Input: part model. Units: mm. Frame: model coordinates. Face numbers are marked on the shaded views. A direction names the side the tool comes from. Round coordinates to 2 decimals unless told otherwise and drop trailing zeros. Loops run counter-clockwise (first coordinate to the right, second up) from the corner with the lowest first, then second, coordinate; pieces in that order, holes last. Notation, with made-up numbers: (-3.75, 25.5) -> (24.25, 25.5) arc R24 cw to (24.25, 50.5) -> close; hole circle Ø10 at (-25.75, -5.5). An arc over 180 degrees is marked (long way). Answer as a JSON object with one key per item and string values.
```python
from build123d import *

# Parameters (mm, degrees)
F1_DEPTH = 5
F2_W     = 160
F2_H     = 2.5
F3_DEPTH = 25
F4_W     = 35
F4_H     = 30
F5_DEPTH = 4
F6_W     = 35
F6_H     = 30
F7_DEPTH = 4
F8_W     = 168
F8_H     = 35
F9_DEPTH = 4


with BuildPart() as f1:
    # F0 (on Top) → F1 (new body)
    with BuildSketch(Plane.XY):
        with BuildLine():
            Line((-60.891874, 20), (-60.891874, 0))
            Line((-60.891874, 0), (-60.891874, -15))
            Line((-60.891874, -15), (99.108126, -15))
            Line((99.108126, -15), (99.108126, 0))
            Line((99.108126, 0), (99.108126, 20))
            Line((99.108126, 20), (95.108126, 20))
            ThreePointArc((95.108126, 20), (79.108126, 4), (63.108126, 20))
            Line((63.108126, 20), (55.108126, 20))
            ThreePointArc((55.108126, 20), (39.108126, 4), (23.108126, 20))
            Line((23.108126, 20), (15.108126, 20))
            ThreePointArc((15.108126, 20), (-0.891874, 4), (-16.891874, 20))
            Line((-16.891874, 20), (-24.891874, 20))
            ThreePointArc((-24.891874, 20), (-40.891874, 4), (-56.891874, 20))
            Line((-56.891874, 20), (-60.891874, 20))
        make_face()
    extrude(amount=F1_DEPTH)

    # F2 (on face) → F3 (join)
    with BuildSketch(Plane.XY.offset(5)):
        with Locations((19.108126, -13.75)):
            Rectangle(F2_W, F2_H)
    extrude(amount=F3_DEPTH)

    # F4 (on face) → F5 (join)
    with BuildSketch(Plane.YZ.offset(99.108126)):
        with Locations((2.5, 15)):
            Rectangle(F4_W, F4_H)
    extrude(amount=F5_DEPTH)

    # F6 (on face) → F7 (join)
    with BuildSketch(Plane(origin=(-60.891874, 0, 0), x_dir=(0, -1, 0), z_dir=(-1, 0, 0))):
        with Locations((-2.5, 15)):
            Rectangle(F6_W, F6_H)
    extrude(amount=F7_DEPTH)

    # F8 (on face) → F9 (join)
    with BuildSketch(Plane.XY.offset(30)):
        with Locations((19.108126, 2.5)):
            Rectangle(F8_W, F8_H)
    extrude(amount=F9_DEPTH)


solid = f1.part
```
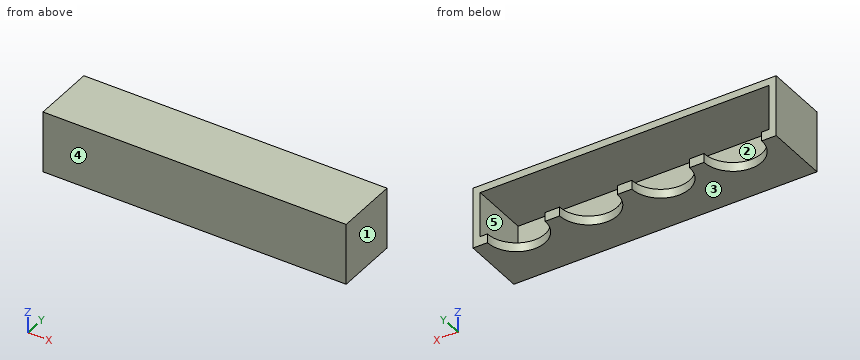
1) Section B-B, the plane x = 21. Output: boundary loops of the cut face in (y, z).
Output:
{"outline": "(-15, 0) -> (20, 0) -> (20, 5) -> (-12.5, 5) -> (-12.5, 30) -> (20, 30) -> (20, 34) -> (-15, 34) -> close"}
2) Reachability of the marked faces 4 and 5 from +Z, -Z, +X, -X, +Y, -Y: full face, straight path, thin tool, end or side. Return the list, or none.
Output:
{"face 4": "+Z, -Z, +X, -X, -Y", "face 5": "+Y"}
3) Section C-C, the plane y = 8. Output: boundary loops of the cut face in (x, z), plus the area to 3 significant figures.
Output:
{"outline": "(-64.89, 0) -> (-51.47, 0) -> (-51.47, 5) -> (-60.89, 5) -> (-60.89, 30) -> (99.11, 30) -> (99.11, 5) -> (89.69, 5) -> (89.69, 0) -> (103.11, 0) -> (103.11, 34) -> (-64.89, 34) -> close; (-30.31, 0) -> (-11.47, 0) -> (-11.47, 5) -> (-30.31, 5) -> close; (9.69, 0) -> (28.53, 0) -> (28.53, 5) -> (9.69, 5) -> close; (49.69, 0) -> (68.53, 0) -> (68.53, 5) -> (49.69, 5) -> close", "area": "1,290 mm^2"}
4) Section A-A, the plane y = -10. Output: boundary loops of the cut face in (x, z), plus the area to 3 significant figures.
Output:
{"outline": "(-64.89, 0) -> (103.11, 0) -> (103.11, 34) -> (-64.89, 34) -> close; hole (-60.89, 5) -> (99.11, 5) -> (99.11, 30) -> (-60.89, 30) -> close", "area": "1,710 mm^2"}
5) Draft query along Z for the marked faces 1, 2 and 3. Return one class per face: +Z half, -Z half, draft (parallel to the pull), parting line (faces both ways), or undercut.
Output:
{"face 1": "draft", "face 2": "undercut", "face 3": "-Z half"}
6) Ray query, probe 1 along Z at (x, y) = (-52, 0.5); probe 2 along X at (y, z) = (2.5, 24.5); probe 3 along Z at (x, y) = (81, 6). Return the intervals inside material, ascending.
Output:
{"probe 1": "z = 0 to 5, 30 to 34", "probe 2": "x = -64.89 to -60.89, 99.11 to 103.11", "probe 3": "z = 30 to 34"}
7) Section D-D, the plane z = 24.5. Output: boundary loops of the cut face in (x, y), plus the area to 3 significant figures.
Output:
{"outline": "(-64.89, -15) -> (103.11, -15) -> (103.11, 20) -> (99.11, 20) -> (99.11, -12.5) -> (-60.89, -12.5) -> (-60.89, 20) -> (-64.89, 20) -> close", "area": "680 mm^2"}
8) Contact query for flat-ended pins moving along their axis: P1, Ø3, axis at x = -45, z = 18.5, coming from the +Y side; P2, Ø2, axis at x = -14, z = 29.5, coming from the +Y side; P3, Ø3, axis at x = 41.5, y = 12.5, coming from the -Z side. Output: stop coordinate, or through.
Output:
{"P1": "stops at y = -12.5", "P2": "stops at y = 20", "P3": "stops at z = 30"}
